Autodesk Inventor part; units mm, degrees
ref_plane "YZ Plane" through (0, 0, 0) normal (1, 0, 0) x (0, 1, 0)
ref_plane "XZ Plane" through (0, 0, 0) normal (0, 1, 0) x (-1, 0, 0)
ref_plane "XY Plane" through (0, 0, 0) normal (0, 0, 1) x (1, 0, 0)
sketch "Sketch2" plane through (0, 0, 0) normal (0, 0, 1) x (1, 0, 0)
  line L0 (0, 12.7947) -> (11.0805, 6.3973)
  line L1 (11.0805, 6.3973) -> (11.0805, -6.3973)
  line L2 (11.0805, -6.3973) -> (0, -12.7947)
  line L3 (0, -12.7947) -> (-11.0805, -6.3973)
  line L4 (-11.0805, -6.3973) -> (-11.0805, 6.3973)
  line L5 (-11.0805, 6.3973) -> (0, 12.7947)
  circle A0 centre (0, 0) radius 6
  dimension "d0" = 12
extrude "Extrusion1" add sketch "Sketch2" along normal blind 12
sketch "Sketch5" plane through (0, 0, 0) normal (1, 0, 0) x (0, 1, 0)
  line L0 (13.8205, 4.649) -> (13.8205, -1.691)
  line L1 (13.8205, -1.691) -> (9.8308, -1.691)
  line L2 (9.8308, -1.691) -> (13.8205, 4.649)
  line L3 (0, -4.894) -> (0, 14.8157)
  point P0 (0, 0)
revolve "Revolution1" cut sketch "Sketch5" angle 360 about axis through (0, 0, 0) along (0, 0, 1)
properties part number "nut M12"
The model under review builds one solid part; all positions refer to its coordinate system, in mm. Round coordinates to 2 decimals unless told otherwise and drop trailing zeros. Loops run counter-clockwise (first coordinate to the right, second up) from the corner with the lowest first, then second, coordinate; pieces in that order, holes last. Notation, with made-up numbers: (6.25, 89) -> (48.25, 89) arc R13 cw to (48.25, 97) -> close; hole circle Ø11 at (-25.5, 25). An arc over 180 degrees is marked (long way). One line per question, with ' | ' between items. Start each with the question number.
Item 1: Wall thickness on line 1 along X through (y, z) = (1.25, 6.5); line 2 along Y through (x, z) = (-3.75, 2.5); line 3 along Y through (x, z) = (-3.25, 2): over which ranges is each line inside the solid? List them lowest first. Write a range as [from, to].
Item 2: Add section B-B, the plane z = 3.75. Write out the cut boundary in (x, y), then the cut area to 3 significant figures.
Item 3: Add section A-A, the plane y = 0. Write out the cut boundary in (x, z).
Item 4: For pin 1 (2 mm diameter, centred on y = 7.5, z = 9.5, fed in from +X); pin 2 (4 mm diameter, centred on x = 3, z = 10.5, fed in from -Y); pin 3 (7 mm diameter, centred on x = 0, y = 0, fed in from +Z), all flat-tipped, find the tip position at first contact; note any pin that passes through.
Return value:
1) line 1: x = [-11.08, -5.87], [5.87, 11.08] | line 2: y = [-10.63, -4.68], [4.68, 10.63] | line 3: y = [-10.92, -5.04], [5.04, 10.92]
2) outline: (-11.08, -6.4) -> (0, -12.79) -> (11.08, -6.4) -> (11.08, 6.4) -> (0, 12.79) -> (-11.08, 6.4) -> close; hole circle Ø12 at (0, 0) | area: 312 mm2
3) outline: (-11.08, 0.29) -> (-10.89, 0) -> (-6, 0) -> (-6, 12) -> (-11.08, 12) -> close; (6, 0) -> (10.89, 0) -> (11.08, 0.29) -> (11.08, 12) -> (6, 12) -> close
4) pin 1: stops at x = 10.9 | pin 2: stops at y = -12.22 | pin 3: passes through
